```python
from build123d import *

# Parameters (mm, degrees)
BOSS_EXTRUDE1_DEPTH = 250
CUT_EXTRUDE1_DEPTH  = 250


with BuildPart() as part:
    # Sketch2 → Boss-Extrude1 (new body)
    with BuildSketch(Plane(origin=(0, 0, 0), x_dir=(0, 0, -1), z_dir=(1, 0, 0))):
        Polygon((-25, -75), (-25, -25), (-75, -25), (-75, 25), (75, 25), (75, -25), (25, -25), (25, -75), (225, -75), (225, 75), (-225, 75), (-225, -75), align=None)
    extrude(amount=-BOSS_EXTRUDE1_DEPTH)

    # Sketch3 → Cut-Extrude1 (cut)
    with BuildSketch(Plane(origin=(0, 75, 0), x_dir=(1, 0, 0), z_dir=(0, 1, 0))):
        Polygon((-100, 225), (-100, 175), (-50, 175), (-50, 125), (-200, 125), (-200, 175), (-150, 175), (-150, 225), align=None)
    extrude(amount=-CUT_EXTRUDE1_DEPTH, mode=Mode.SUBTRACT)


solid = part.part
```
Part model, mm, in its own coordinate system. A direction names the side the tool comes from. Give positions to 0.01 mm unless a question says otherwise; leave off trailing zeros. Order: outer loops, then holes, each group sorted by start corner. A loop starts at its lowest first (then second) coordinate and runs counter-clockwise, first axis right, second up. Notation, with made-up numbers: (33.5, 44.5) - (70.5, 44.5) arc R29 ccw to (70.5, 79.5) - close; hole circle Ø2 at (3.25, -7.75). An arc over 180 degrees is marked (long way). Use one line per item in the form item = value.
Item 1: Probe probe 1 along Z at (x, y) = (-155.5, 18); probe 2 along Z at (x, y) = (-83.5, -64.5); probe 3 along X at (y, z) = (-21, -169). List the from-to ranges inside material, lowest first. Write a range as from..to.
Solution:
probe_1 = -225..-175, -125..-75, 75..225
probe_2 = -225..-175, -125..-25, 25..225
probe_3 = -250..-200, -50..0
Item 2: Slice it at C-C on z = -136.5. Give the cut face in (x, y).
Solution:
outline = (-250, -75) - (-200, -75) - (-200, 75) - (-250, 75) - close; (-50, -75) - (0, -75) - (0, 75) - (-50, 75) - close
Item 3: Two-plate mould, pull along Z, no slides. Class faces 5 (the face through (-123, 0, -75)), 6 (the face through (-150, 1, -200)), 7 (the face through (-199, -1, -225)): released by +Z, released by -Z, zero draft, split by the parting line, or undercut.
Solution:
face_5 = undercut
face_6 = zero draft
face_7 = released by -Z
Item 4: Slice it at D-D on y = 58.5. Give the cut face in (x, z), and give its area (4 significant figures).
Solution:
outline = (-250, -225) - (-150, -225) - (-150, -175) - (-200, -175) - (-200, -125) - (-50, -125) - (-50, -175) - (-100, -175) - (-100, -225) - (0, -225) - (0, 225) - (-250, 225) - close
area = 102,500 mm2
Item 5: Which spindle directions (+Z, -Z, +X, -X, +Y, -Y) get a long thin tool onto all of the face, cutting with end or side? Do faces 1 (the face through (-100, 1, -200)), 2 (the face through (-123, 25, 1)), 3 (the face through (-123, -50, 25)), 4 (the face through (-175, 1, -175)). Say none if no direction does.
Solution:
face_1 = -Z, +Y, -Y
face_2 = +X, -X
face_3 = +X, -X, -Y
face_4 = +Y, -Y
Item 6: Pin check, flat tip, straight feed: pin 1 Ø15 at (x, y) = (-146, -3) entering from -Z. Stop position of the tip, or through.
Solution:
pin_1 = -225
Item 7: Slice it at A-A on y = -62.5. Give the cut face in (x, z).
Solution:
outline = (-250, -225) - (-150, -225) - (-150, -175) - (-200, -175) - (-200, -125) - (-50, -125) - (-50, -175) - (-100, -175) - (-100, -225) - (0, -225) - (0, -25) - (-250, -25) - close; (-250, 25) - (0, 25) - (0, 225) - (-250, 225) - close
Item 8: Slice it at B-B on x = -193.5. Give the cut face in (y, z), and give its area (3 significant figures).
Solution:
outline = (-75, -225) - (75, -225) - (75, -175) - (-75, -175) - close; (-75, -125) - (75, -125) - (75, 225) - (-75, 225) - (-75, 25) - (-25, 25) - (-25, 75) - (25, 75) - (25, -75) - (-25, -75) - (-25, -25) - (-75, -25) - close
area = 50,000 mm2
